Can you work these out from the drawing? Everything is in mm from the part's minimum corner. A direction names the side the tool comes from. Coordinates: 2 decimals unless noted, no trailing zeros. Loops run counter-clockwise (first coordinate to the right, second up) from the corner with the lowest first, then second, coordinate; pieces in that order, holes last.
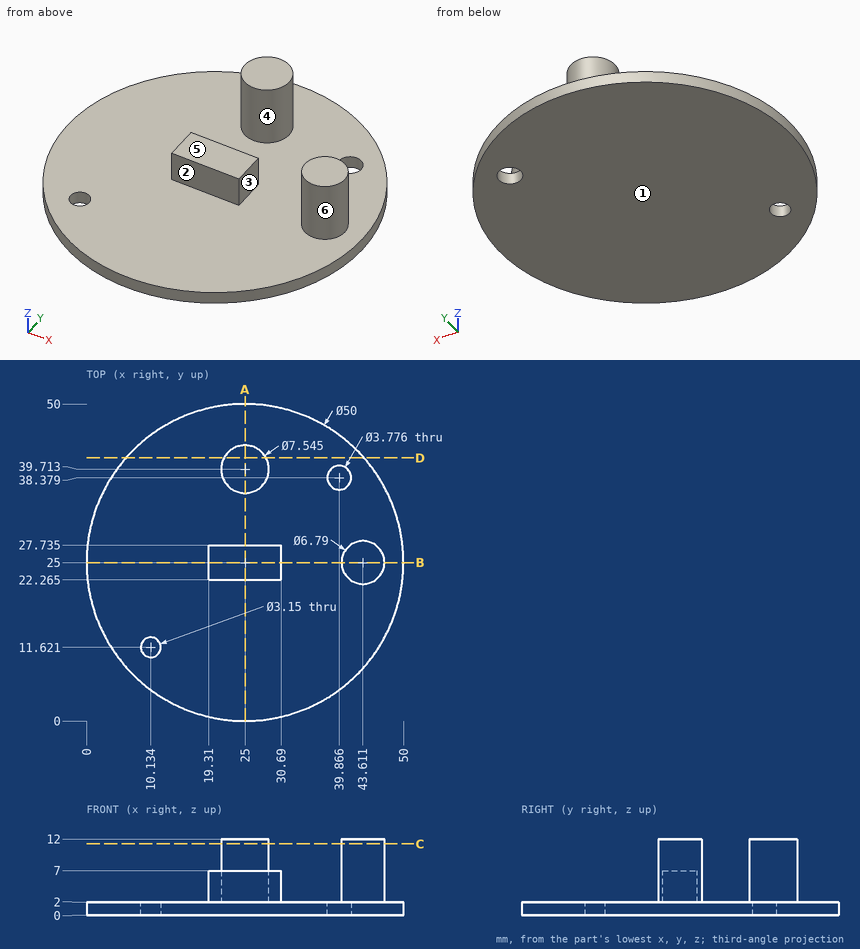
Item 1: Suppose I cut it at A-A, the plane x = 25. Please give me the cut outline in (y, z) (1 decimal), plus the area to 3 significant figures.
Results are:
outline: (0, 0) - (50, 0) - (50, 2) - (43.5, 2) - (43.5, 12) - (35.9, 12) - (35.9, 2) - (27.7, 2) - (27.7, 7) - (22.3, 7) - (22.3, 2) - (0, 2) - close
area: 203 mm2
Item 2: Suppose I cut it at D-D, the plane y = 41.5. Please give me the cut outline in (x, z).
Results are:
outline: (6.22, 0) - (43.78, 0) - (43.78, 2) - (28.32, 2) - (28.32, 12) - (21.68, 12) - (21.68, 2) - (6.22, 2) - close
Item 3: On a 3-axis mill with a long thin cutter (end or side, diameter ignored), from which of +Z, -Z, +X, -X, +Y, -Y can I reach the whole of each face in a straight line? I mean the marked faces 1, 2 and 3. Say none if no direction works.
Results are:
face 1: -Z, +X, -X, +Y, -Y
face 2: +Z, -X, -Y
face 3: +Z, +Y, -Y
Item 4: Suppose I cut it at B-B, the plane y = 25. Please give me the cut outline in (x, z) (1 decimal), plus the area to 3 significant figures.
Results are:
outline: (0, 0) - (50, 0) - (50, 2) - (47, 2) - (47, 12) - (40.2, 12) - (40.2, 2) - (30.7, 2) - (30.7, 7) - (19.3, 7) - (19.3, 2) - (0, 2) - close
area: 225 mm2
Item 5: I need wall thicknesses on line 1 along Z through (x, y) = (28.5, 4.5); line 2 along Y through (x, z) = (29.5, 6.75) (1 decimal); line 3 along Z through (x, y) = (23, 24). Which ranges of each line are inside material? Lowest first, please.
Results are:
line 1: z = 0 to 2
line 2: y = 22.3 to 27.7
line 3: z = 0 to 7
Item 6: We'd pull the mould along Y, two halves only. Please class the marked faces 4, 5 and 6: +Y half, -Y half, draft (parallel to the pull), parting line (faces both ways), or undercut.
Results are:
face 4: undercut
face 5: draft
face 6: parting line
Item 7: Suppose I cut it at C-C, the plane z = 11.25. Please give me the cut outline in (x, y) (1 decimal).
Results are:
outline: circle Ø7.5 at (25, 39.7); circle Ø6.8 at (43.6, 25)
Item 8: I'm going to push flat-ended pins straight in: P1, Ø2.5, axis at y = 24, z = 5, coming from the -X side; P2, Ø5.5, axis at y = 26, z = 5.5, coming from the +X side; P3, Ø2.5, axis at x = 22.5, z = 4.5, coming from the +Y side. Where does each tip first touch, or does it pass through?
Results are:
P1: stops at x = 19.31
P2: stops at x = 47.01
P3: stops at y = 43.27
